from build123d import *

# Parameters (mm, degrees)
SKETCH1_R                = 5.85
BOSS_EXTRUDE1_DEPTH      = 100
SKETCH2_R                = 7.8
BOSS_EXTRUDE2_DEPTH      = 30
BOSS_EXTRUDE3_DEPTH      = 3
BOSS_EXTRUDE3_DEPTH_BACK = 3
SKETCH3_W                = 1.478387163
SKETCH3_H                = 20


with BuildPart() as part:
    # Sketch1 → Boss-Extrude1 (new body)
    with BuildSketch(Plane(origin=(0, 0, 0), x_dir=(1, 0, 0), z_dir=(0, 1, 0))):
        with Locations(Location((0, 0, 0), (0, 0, 270))):
            Circle(SKETCH1_R)
    extrude(amount=BOSS_EXTRUDE1_DEPTH)

    # Sketch2 → Boss-Extrude2 (add)
    with BuildSketch(Plane(origin=(0, 100, 0), x_dir=(1, 0, 0), z_dir=(0, 1, 0))):
        with Locations(Location((0, 0, 0), (0, 0, 270))):
            Circle(SKETCH2_R)
    extrude(amount=BOSS_EXTRUDE2_DEPTH)

    # Sketch3 → Boss-Extrude3 (add, two sides: drawn at the far end of the back side and taken through both)
    with BuildSketch(Plane.XY.offset(-BOSS_EXTRUDE3_DEPTH_BACK)):
        with Locations((0.739193582, -10)):
            Rectangle(SKETCH3_W, SKETCH3_H)
        with Locations((-0.739193582, -10)):
            Rectangle(SKETCH3_W, SKETCH3_H)
        with BuildLine():
            Line((1.478387163, -20), (-1.478387163, -20))
            ThreePointArc((-1.478387163, -20), (0, -21.478387163), (1.478387163, -20))
        make_face()
    extrude(amount=BOSS_EXTRUDE3_DEPTH + BOSS_EXTRUDE3_DEPTH_BACK)


solid = part.part
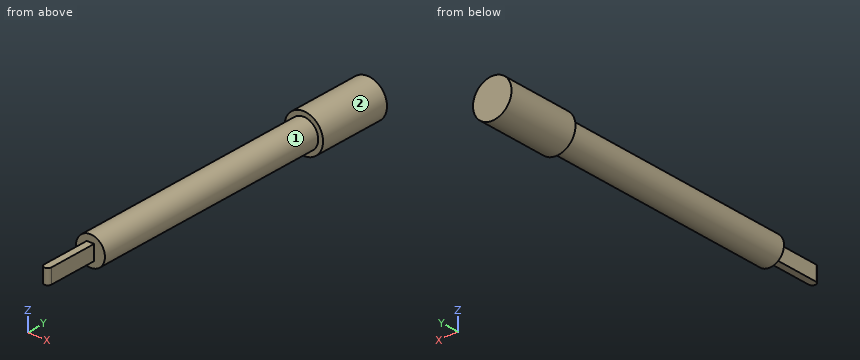
Could you check a few things on this model? Use its own coordinates, in mm. Face numbers are marked on the shaded views. A direction names the side the tool comes from. Give positions to 0.01 mm unless a question says otherwise; leave off trailing zeros. Order: outer loops, then holes, each group sorted by start corner. A loop starts at its lowest first (then second) coordinate and runs counter-clockwise, first axis right, second up. Notation, with made-up numbers: (-1.5, 53) - (10.5, 53) arc R32 cw to (10.5, 81) - close; hole circle Ø2 at (68.25, 61). An arc over 180 degrees is marked (long way). One line per item, written item: value. Start each with the question number.
1. Imagine slicing it at B-B on z = 0. List the corners of the cut face in (x, y) for me, plus the area to 3 significant figures.
2. Imagine slicing it at C-C on y = 119. List the corners of the cut face in (x, z) for me.
3. If I drill on probe 1 along Y at (x, z) = (-3.5, 4.75); probe 2 along X at (y, z) = (-13, 2.75); probe 3 along Y at (x, z) = (3.25, -0.5), over which ranges is the centre line in solid material (lowest first)?
4. Imagine slicing it at A-A on x = 0. List the corners of the cut face in (y, z) for me, plus the area to 3 significant figures.
5. Imagine slicing it at D-D on y = 37.5. List the corners of the cut face in (x, z) for me, plus the area to 3 significant figures.
6. For P1, Ø3, axis at x = 3.5, y = 84, coming from the +Z side; P2, Ø4, axis at x = -6, y = 68.5, coming from the -Z side; P3, Ø1.5, axis at x = 0, y = -7, coming from the -Z side, each with a flat end and sliding along its axis, tell me the tip position at first contact or that it passes through.
7. For the marked faces 1 and 2, which set-ups out of +Z, -Z, +X, -X, +Y, -Y let a thin tool reach every point of the face, with its end or its side?
Values:
1. outline: (-7.8, 100) - (-5.85, 100) - (-5.85, 0) - (-1.48, 0) - (-1.48, -20) arc R1.48 ccw to (1.48, -20) - (1.48, 0) - (5.85, 0) - (5.85, 100) - (7.8, 100) - (7.8, 130) - (-7.8, 130) - close
1. area: 1,700 mm²
2. outline: circle Ø15.6 at (0, 0)
3. probe 1: 100 to 130
3. probe 2: -1.48 to 1.48
3. probe 3: 0 to 130
4. outline: (-21.48, -3) - (0, -3) - (0, -5.85) - (100, -5.85) - (100, -7.8) - (130, -7.8) - (130, 7.8) - (100, 7.8) - (100, 5.85) - (0, 5.85) - (0, 3) - (-21.48, 3) - close
4. area: 1,770 mm²
5. outline: circle Ø11.7 at (0, 0)
5. area: 108 mm²
6. P1: z = 5.5
6. P2: z = -4.27
6. P3: z = -3
7. face 1: -Y
7. face 2: +Y, -Y
